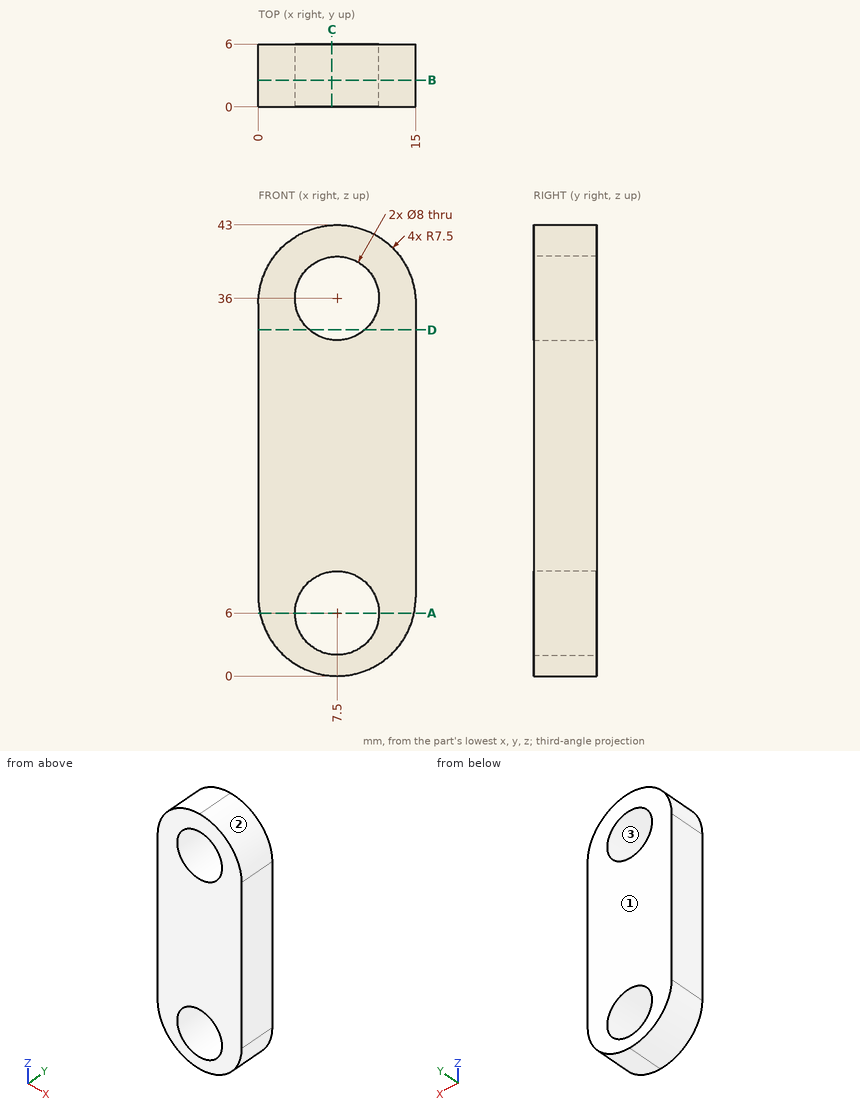
Geometry: see drawing. Coordinates: mm, zero at the bounding-box minimum. Give positions to 0.01 mm unless a question says otherwise; leave off trailing zeros. Order: outer loops, then holes, each group sorted by start corner. A loop starts at its lowest first (then second) coordinate and runs counter-clockwise, first axis right, second up. Notation, with made-up numbers: M 76,-13 L 101,-13 A29 cw 101,18 Z; hole C 28,-2 d10. An arc over 180 degrees is marked long. Answer as a JSON object with one key per item and string values.
1. Cut plane A-A, the plane z = 6. Output: boundary loops of the cut face in (x, y).
Result sheet:
{"outline": "M 0.15,0 L 3.5,0 L 3.5,6 L 0.15,6 Z; M 11.5,0 L 14.85,0 L 14.85,6 L 11.5,6 Z"}
2. First-contact query: P1, Ø5, axis at x = 7.5, z = 36, coming from the -Y side. Flat tip, straight axial feed; report the tip coordinate or a pass-through.
Result sheet:
{"P1": "through"}
3. Ray query, line 1 (Z direction, x = 4.25, y = 1.45); line 2 (X direction, y = 3.9, z = 36); line 3 (X direction, y = 2.35, z = 6). Return the intervals inside material, ascending. Write a range as [from, to].
Result sheet:
{"line 1": "[0.74, 3.67], [8.33, 33.67], [38.33, 42.26]", "line 2": "[0.02, 3.5], [11.5, 14.98]", "line 3": "[0.15, 3.5], [11.5, 14.85]"}
4. Cut plane D-D, the plane z = 33. Output: boundary loops of the cut face in (x, y).
Result sheet:
{"outline": "M 0,0 L 4.85,0 L 4.85,6 L 0,6 Z; M 10.15,0 L 15,0 L 15,6 L 10.15,6 Z"}
5. Pull-direction query (X, two-part tool) for the marked faces 1, 2 and 3; classes: +X half, -X half, draft (parallel to the pull), parting line (faces both ways), or undercut.
Result sheet:
{"face 1": "draft", "face 2": "+X half", "face 3": "undercut"}
6. Cut plane B-B, the plane y = 2.55. State how many separate pieces and enclosed holes the cut face has, and give its area (3 significant figures).
Result sheet:
{"separate pieces": "1", "enclosed holes": "2", "area": "496 mm²"}
7. Cut plane C-C, the plane x = 7. Output: boundary loops of the cut face in (y, z).
Result sheet:
{"outline": "M 0,0.02 L 6,0.02 L 6,2.03 L 0,2.03 Z; M 0,9.97 L 6,9.97 L 6,32.03 L 0,32.03 Z; M 0,39.97 L 6,39.97 L 6,42.98 L 0,42.98 Z"}
